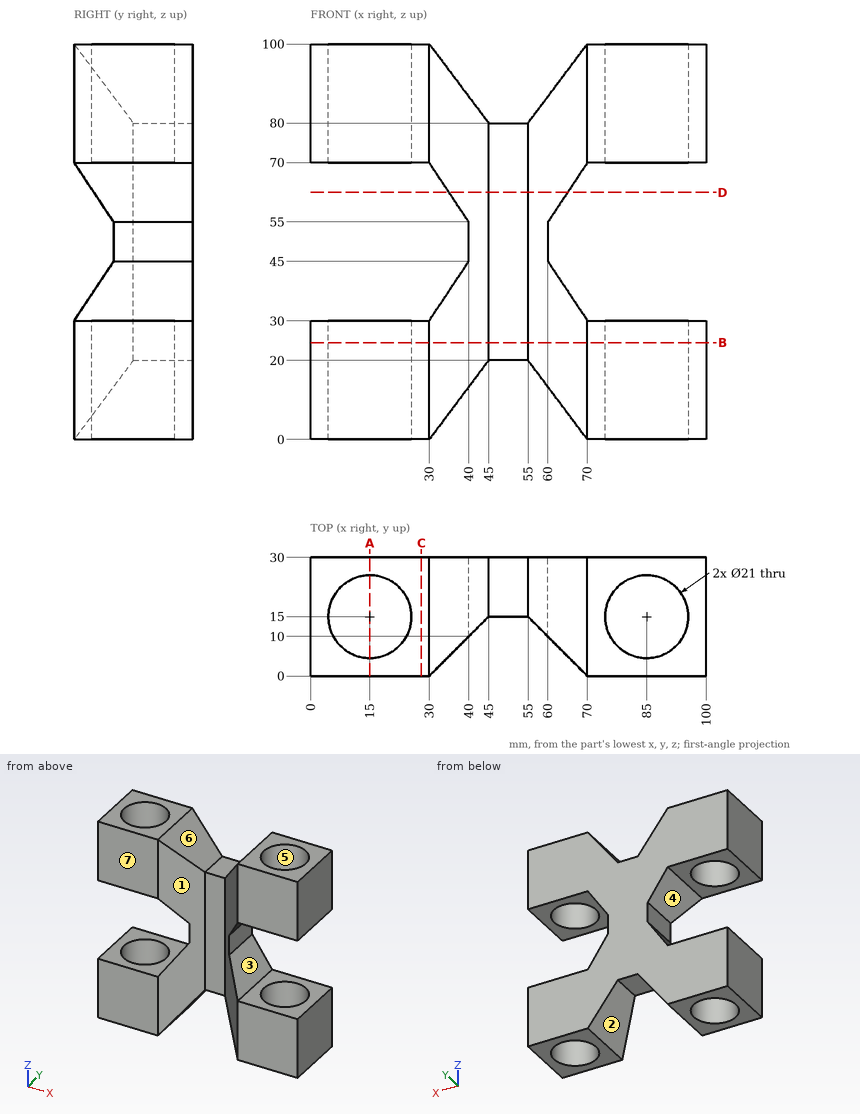
For this review, use the dimensioned drawing (mm, ordinates from the lowest corner) and the shaded views. A direction names the side the tool comes from. Coordinates: 2 decimals unless noted, no trailing zeros. Order: outer loops, then holes, each group sorted by start corner. A loop starts at its lowest first (then second) coordinate and runs counter-clockwise, first axis right, second up. Notation, with made-up numbers: (53.25, -33.75) - (107.25, -33.75) arc R23 ccw to (107.25, 4.25) - close; hole circle Ø1 at (45.25, -38). An arc over 180 degrees is marked (long way). Answer as a JSON object with one key per item and string values. Group by question number.
1. For probe 1 along Y at (x, z) = (15, 7.5); probe 2 along X at (y, z) = (15.25, 27.5); probe 3 along X at (y, z) = (13, 91.5) (3 decimals), list the stretches that pass through material, from the lowest coordinate up.
2. Clearance check with flat-ended pins moving along their axes: P1, Ø3, axis at x = 47.5, y = 19.5, coming from the +Z side; P2, Ø3, axis at y = 12.5, z = 69.5, coming from the -X side; P3, Ø6, axis at x = 19, z = 35.5, coming from the -Y side; P4, Ø5, axis at x = 49.5, z = 40.5, coming from the -Y side. State where each tip first meets the part, or that it passes through.
3. We need section A-A on x = 15. State the section outline as (y, z) points, then the cut area to 3 significant figures.
4. We need section C-C on x = 28. State the section outline as (y, z) points, then the cut area to 3 significant figures.
5. We need section D-D on z = 62.5. State the section outline as (x, y) points, then the cut area to 3 significant figures.
6. For the marked faces 1, 2, 3 and 4, list the 3-axis set-ups (+Z, -Z, +X, -X, +Y, -Y) from which the entire face can be reached by the end or side of a thin tool; tool diameter is ignored.
7. The part is to be moulded in two halves that separate along Y. For the marked faces 5, 6 and 7, say which applies: pulls with the +Y half, pulls with the -Y half, needs draft (parallel to the pull), parting line crosses it, or undercut.
8. We need section B-B on z = 24.5. State the section outline as (x, y) points, then the cut area to 3 significant figures.
Final values:
{
 "1": {"probe 1": "0 to 4.5, 25.5 to 30", "probe 2": "0 to 4.5, 25.5 to 74.5, 95.5 to 100", "probe 3": "0 to 4.692, 25.308 to 36.375, 63.625 to 74.692, 95.308 to 100"},
 "2": {"P1": "z = 80", "P2": "x = 0", "P3": "through", "P4": "y = 15"},
 "3": {"outline": "(0, 0) - (4.5, 0) - (4.5, 30) - (0, 30) - close; (0, 70) - (4.5, 70) - (4.5, 100) - (0, 100) - close; (25.5, 0) - (30, 0) - (30, 30) - (25.5, 30) - close; (25.5, 70) - (30, 70) - (30, 100) - (25.5, 100) - close", "area": "540 mm²"},
 "4": {"outline": "(0, 0) - (30, 0) - (30, 30) - (0, 30) - close; (0, 70) - (30, 70) - (30, 100) - (0, 100) - close", "area": "1,800 mm²"},
 "5": {"outline": "(35, 5) - (45, 15) - (55, 15) - (65, 5) - (65, 30) - (35, 30) - close", "area": "550 mm²"},
 "6": {"face 1": "+Z, -Z, -Y", "face 2": "-Z, +Y, -Y", "face 3": "+X, +Y, -Y", "face 4": "-X, +Y, -Y"},
 "7": {"face 5": "undercut", "face 6": "needs draft", "face 7": "pulls with the -Y half"},
 "8": {"outline": "(0, 0) - (30, 0) - (45, 15) - (55, 15) - (70, 0) - (100, 0) - (100, 30) - (0, 30) - close; hole circle Ø21 at (15, 15); hole circle Ø21 at (85, 15)", "area": "1,930 mm²"}
}
